from build123d import *

# Parameters (mm, degrees)
SKETCH1_W           = 12.7
SKETCH1_H           = 19.05
BOSS_EXTRUDE1_DEPTH = 7.62
SKETCH3_R           = 1.75
CUT_EXTRUDE1_DEPTH  = 22.2885
SKETCH4_R           = 2
CUT_EXTRUDE2_DEPTH  = 22.2885


with BuildPart() as part:
    # Sketch1 → Boss-Extrude1 (new body)
    with BuildSketch(Plane.YZ):
        Rectangle(SKETCH1_W, SKETCH1_H)
    extrude(amount=BOSS_EXTRUDE1_DEPTH)

    # Sketch3 → Cut-Extrude1 (cut)
    with BuildSketch(Plane.XZ.offset(6.35)):
        with Locations(Location((4.36625, 0, 0), (0, 0, 270))):
            Circle(SKETCH3_R)
    extrude(amount=-CUT_EXTRUDE1_DEPTH, mode=Mode.SUBTRACT)

    # Sketch4 → Cut-Extrude2 (cut)
    with BuildSketch(Plane.YZ.offset(7.62)):
        with Locations(Location((2.54, 4.7625, 0), (0, 0, 270))):
            Circle(SKETCH4_R)
        with Locations(Location((-2.54, -4.7625, 0), (0, 0, 270))):
            Circle(SKETCH4_R)
    extrude(amount=-CUT_EXTRUDE2_DEPTH, mode=Mode.SUBTRACT)


solid = part.part
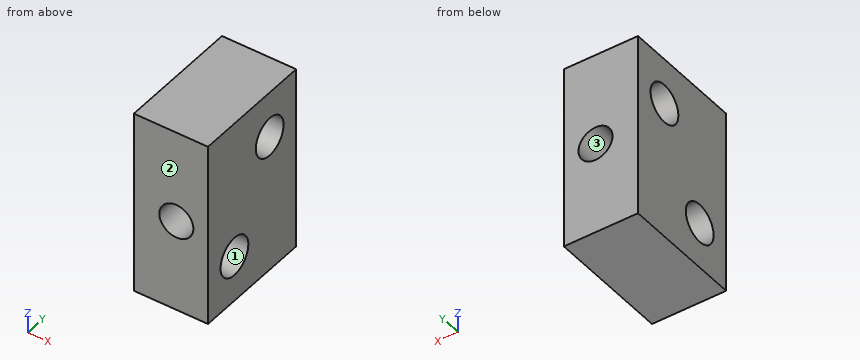
Input: part model. Units: mm. Frame: model coordinates. Face numbers are marked on the shaded views. Coordinates: 2 decimals unless noted, no trailing zeros. Loops run counter-clockwise (first coordinate to the right, second up) from the corner with the lowest first, then second, coordinate; pieces in that order, holes last.
(1) Material intervals for probe 1 along X at (y, z) = (-1.5, 0); probe 2 along Z at (x, y) = (3.5, -4.25) (3 decimals); probe 3 along Y at (x, z) = (4.5, 5.5), sorted ascending.
(2) Section B-B on y = -2. Return the cut outline in (x, z) (3 decimals).
(3) Section C-C on x = 5.5. Count the separate pieces of the cut face and the enclosed holes in it, then the cut area to 3 significant figures.
(4) Pull-direction query (Y, two-part tool) for the marked faces 1, 2 and 3; classes: released by +Y, released by -Y, zero draft, split by the parting line, or undercut.
(5) Section A-A on z = 0. Return the cut outline in (x, y), then the cut area to 3 significant figures.
Data:
1. probe 1: x = 0 to 2.62, 6.12 to 7.62
1. probe 2: z = -9.525 to -5.8, -3.725 to -1.521, 1.521 to 9.525
1. probe 3: y = -6.35 to 0.68, 4.4 to 6.35
2. outline: (0, -9.525) - (7.62, -9.525) - (7.62, -6.688) - (0, -6.688) - close; (0, -2.837) - (7.62, -2.837) - (7.62, 9.525) - (0, 9.525) - close; hole circle Ø3.5 at (4.366, 0)
3. separate pieces: 2
3. enclosed holes: 2
3. area: 183 mm2
4. face 1: undercut
4. face 2: released by -Y
4. face 3: zero draft
5. outline: (0, -6.35) - (2.62, -6.35) - (2.62, 6.35) - (0, 6.35) - close; (6.12, -6.35) - (7.62, -6.35) - (7.62, 6.35) - (6.12, 6.35) - close
5. area: 52.3 mm2
